from build123d import *

# Parameters (mm, degrees)
SKETCH_1_W      = 20
SKETCH_1_H      = 10
SKETCH_1_R      = 1.6
EXTRUDE_1_DEPTH = 24.5
FILLET_1_R      = 5


with BuildPart() as part:
    # ｽｹｯﾁ1 → ﾎﾞｽ - 押し出し1 (new body)
    with BuildSketch(Plane.XY):
        Rectangle(SKETCH_1_W, SKETCH_1_H)
        with Locations((-5, 0.4)):
            Circle(SKETCH_1_R, mode=Mode.SUBTRACT)
        with Locations(Location((5, 0.4, 0), (0, 0, 180))):
            Circle(SKETCH_1_R, mode=Mode.SUBTRACT)
    extrude(amount=EXTRUDE_1_DEPTH)

    # ﾌｨﾚｯﾄ1
    # the kernel refuses this fillet: 5 mm, written as the material it takes off along each edge
    with BuildSketch(Plane(origin=(10, 17.5, 24.5), x_dir=(0, 0, -1), z_dir=(0, -1, 0))) as fillet_1_piece_1:
        with BuildLine():
            CenterArc((FILLET_1_R, -FILLET_1_R), FILLET_1_R, 90, 90)
            Line((0, -FILLET_1_R), (0, 0))
            Line((0, 0), (FILLET_1_R, 0))
        make_face()
    extrude(amount=35, mode=Mode.SUBTRACT)


solid = part.part
Can you work these out from the model? Positions are in its coordinate system, mm. Give positions to 0.01 mm unless a question says otherwise; leave off trailing zeros. Order: outer loops, then holes, each group sorted by start corner. A loop starts at its lowest first (then second) coordinate and runs counter-clockwise, first axis right, second up. Notation, with made-up numbers: M -29,-11 L -24,-11 A18 cw -24,-1 Z; hole C -9.75,11 d7. An arc over 180 degrees is marked long. Use one line per item in the form item = value.
Item 1: If we section it at B-B, the plane y = 0.4: Write out the boundary of the cut face in (x, z).
Values follow:
outline = M -10,0 L -6.6,0 L -6.6,24.5 L -10,24.5 Z; M -3.4,0 L 3.4,0 L 3.4,24.5 L -3.4,24.5 Z; M 6.6,0 L 10,0 L 10,19.5 A5 ccw 6.6,24.24 Z
Item 2: If we section it at A-A, the plane x = -5: Write out the boundary of the cut face in (y, z), and give its area (3 significant figures).
Values follow:
outline = M -5,0 L -1.2,0 L -1.2,24.5 L -5,24.5 Z; M 2,0 L 5,0 L 5,24.5 L 2,24.5 Z
area = 167 mm^2
Item 3: If we section it at D-D, the plane x = 4.25: Write out the boundary of the cut face in (y, z).
Values follow:
outline = M -5,0 L -1.01,0 L -1.01,24.5 L -5,24.5 Z; M 1.81,0 L 5,0 L 5,24.5 L 1.81,24.5 Z
Item 4: If I drill on line 1 along Y through (x, z) = (-5, 18); line 2 along X through (y, z) = (1, 23.25); line 3 along X through (y, z) = (-0.5, 5.5), over which ranges is the centre line in solid material (lowest first)? Write a range as [from, to].
Values follow:
line_1 = [-5, -1.2], [2, 5]
line_2 = [-10, -6.48], [-3.52, 3.52], [6.48, 8.31]
line_3 = [-10, -6.32], [-3.68, 3.68], [6.32, 10]
Item 5: Thinking about a two-plate mould opening in X: for faces 1 (the flat face through (-3, 0, 24.5)), 2 (the cylindrical face through (5, 2, 12)), 3 (the cylindrical face through (8.57, 0.07, 23)), 4 (the cylindrical face through (-6.6, 0.47, 12.08)), which applies, pulls with the +X half, pulls with the -X half, needs draft (parallel to the pull), parting line crosses it, or undercut?
Values follow:
face_1 = needs draft
face_2 = undercut
face_3 = pulls with the +X half
face_4 = undercut
Item 6: If we section it at C-C, the plane z = 4.25: Write out the boundary of the cut face in (x, y), and give its area (3 significant figures).
Values follow:
outline = M -10,-5 L 10,-5 L 10,5 L -10,5 Z; hole C -5,0.4 d3.2; hole C 5,0.4 d3.2
area = 184 mm^2
